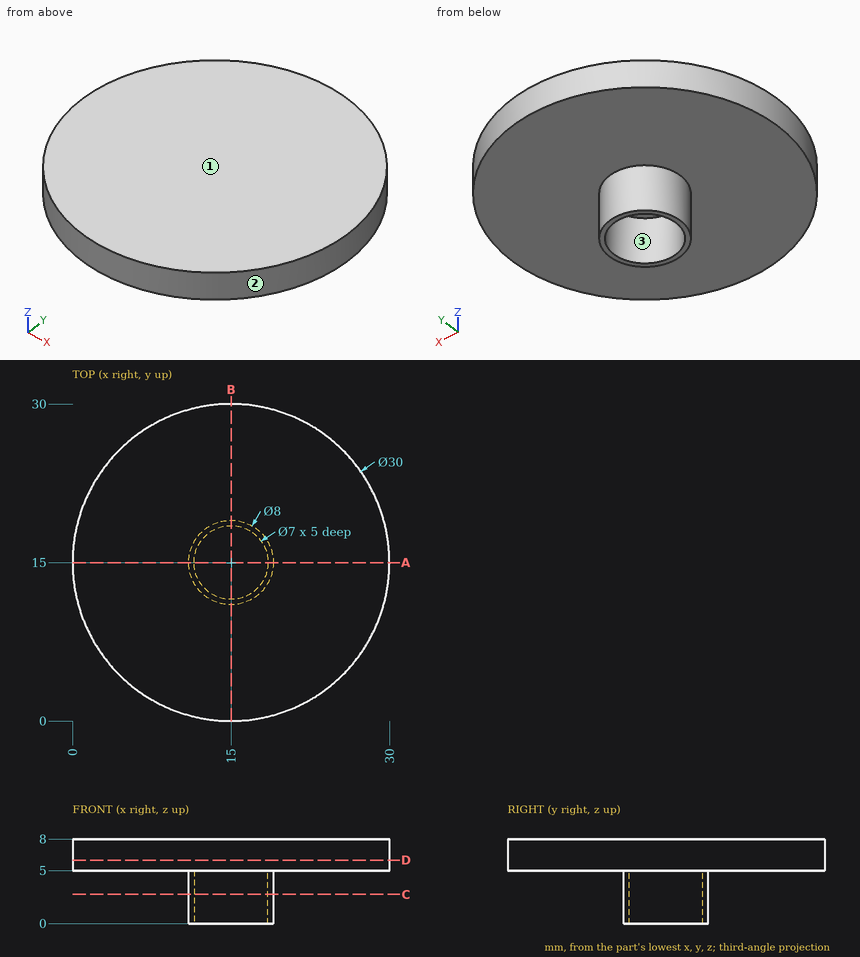
Geometry check sheet. Reference: drawing and pictorial views, mm from the part's lowest x, y, z. Give positions to 0.01 mm unless a question says otherwise; leave off trailing zeros. Loops run counter-clockwise (first coordinate to the right, second up) from the corner with the lowest first, then second, coordinate; pieces in that order, holes last. Notation, with made-up numbers: M 12.25,0 L 36.25,0 A25 cw 36.25,21 Z; hole C 56.5,-31 d8. An arc over 180 degrees is marked long. Use a Markdown table: item, result. Add a question column.
Q1. Scan lines: line 1 along Y through (x, z) = (15, 3.6); line 2 along Z through (x, y) = (15.5, 3); line 3 along X through (y, z) = (13.25, 3.75). Record each from-to range of solid material in increasing order. Write a range as [from, to].
Q2. Sectioned sample at C-C, the plane z = 2.75. Record the cut outline in (x, y).
Q3. Go/stop test with flat-tipped pins: pin 1 (4 mm diameter, centred on x = 16.5, z = 1, fed in from -Y); pin 2 (3 mm diameter, centred on y = 22, z = 2, fed in from -X); pin 3 (6.5 mm diameter, centred on x = 15, y = 15, fed in from -Z); pin 4 (4 mm diameter, centred on x = 18.5, z = 1, fed in from -Y). Record where each tip stops, or that it passes through.
Q4. Mould release check, pull along Y, two halves, no side actions. Record for the marked faces 1, 2 and 3: pulls with the +Y half, pulls with the -Y half, needs draft (parallel to the pull), parting line crosses it, or undercut.
Q5. Sectioned sample at D-D, the plane z = 6. Record the cut outline in (x, y).
Q6. Sectioned sample at A-A, the plane y = 15. Record the cut outline in (x, z), then the cut area to 3 significant figures.
Verdict:
| question | item | result |
|---|---|---|
| 1 | line 1 | [11, 11.5], [18.5, 19] |
| 1 | line 2 | [5, 8] |
| 1 | line 3 | [11.4, 11.97], [18.03, 18.6] |
| 2 | outline | C 15,15 d8; hole C 15,15 d7 |
| 3 | pin 1 | y = 11 |
| 3 | pin 2 | through |
| 3 | pin 3 | z = 5 |
| 3 | pin 4 | y = 11.29 |
| 4 | face 1 | needs draft |
| 4 | face 2 | parting line crosses it |
| 4 | face 3 | undercut |
| 5 | outline | C 15,15 d30 |
| 6 | outline | M 0,5 L 11,5 L 11,0 L 11.5,0 L 11.5,5 L 18.5,5 L 18.5,0 L 19,0 L 19,5 L 30,5 L 30,8 L 0,8 Z |
| 6 | area | 95.0 mm^2 |
